Could you check a few things on this drawing? It's one solid part, dimensions in mm from its lowest x, y, z. A direction names the side the tool comes from. Give positions to 0.01 mm unless a question says otherwise; leave off trailing zeros. Loops run counter-clockwise (first coordinate to the right, second up) from the corner with the lowest first, then second, coordinate; pieces in that order, holes last.
Q1. Suppose I cut it at A-A (x = 35). List the corners of the cut face in (y, z) for me.
Q2. For the marked faces 5 and 6, which set-ups out of +Z, -Z, +X, -X, +Y, -Y let a thin tool reach every point of the face, with its end or its side?
Q3. I need wall thicknesses on probe 1 along X at (y, z) = (36, 17.5) (1 decimal); probe 2 along Y at (x, z) = (17, 25) (1 decimal); probe 3 along Z at (x, y) = (29, 62). Which ranges of each line are inside material? Lowest first, please.
Q4. I'm going to push flat-ended pins straight in: P1, Ø4, axis at x = 57, y = 52, coming from the +Z side; P2, Ø3, axis at y = 38, z = 49, coming from the -X side; P3, Ø12, axis at y = 51.5, z = 47.5, coming from the +X side (1 decimal). Where does each tip first touch, or does it pass through?
Q5. Suppose I cut it at B-B (y = 35). Count the separate pieces of the cut face and the enclosed holes in it, and give its area (3 significant figures).
Q6. Thinking about a two-plate mould opening in X: for the marked faces 1, 2, 3 and 4, which applies, pulls with the +X half, pulls with the -X half, needs draft (parallel to the pull), parting line crosses it, or undercut?
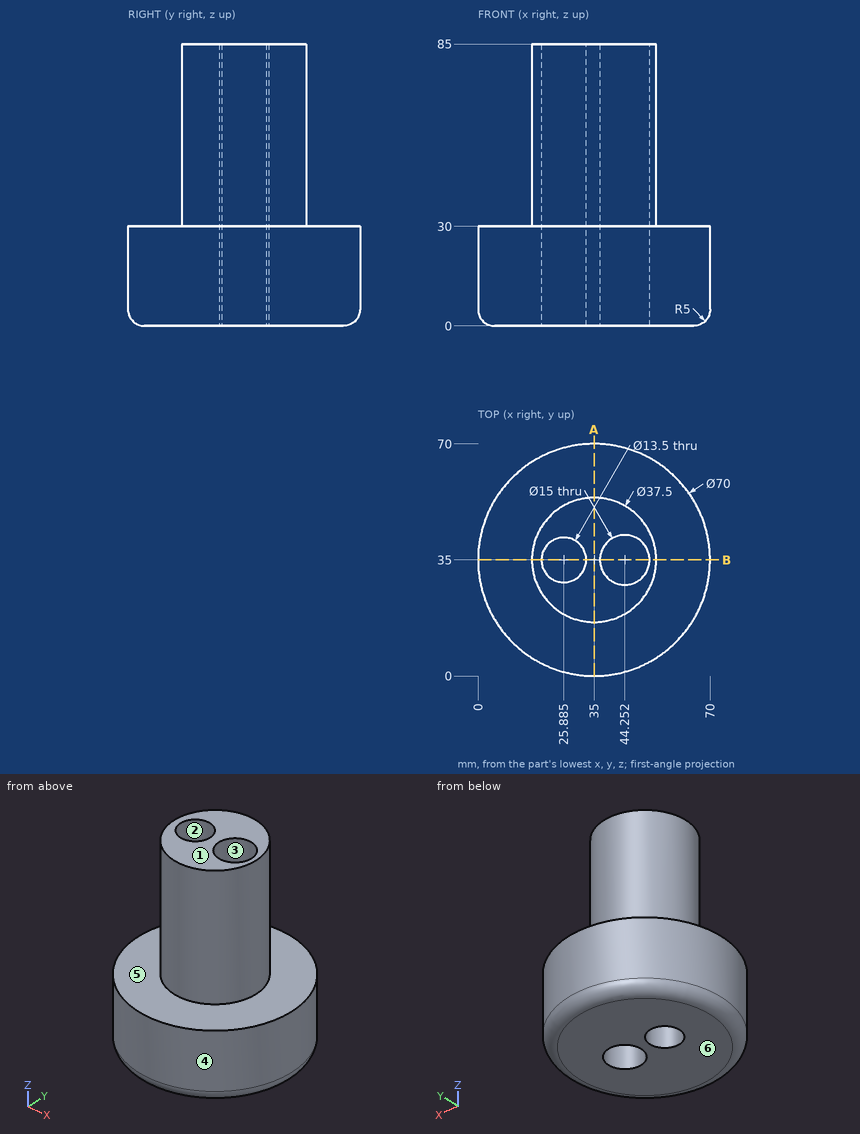
Solutions:
1. outline: (0, 5) arc R5 ccw to (5, 0) - (65, 0) arc R5 ccw to (70, 5) - (70, 30) - (53.75, 30) - (53.75, 85) - (16.25, 85) - (16.25, 30) - (0, 30) - close
2. face 5: +Z
2. face 6: -Z, +X, -X, +Y, -Y
3. probe 1: x = 0 to 19.2, 32.6 to 36.8, 51.7 to 70
3. probe 2: y = 5 to 65
3. probe 3: z = 0 to 30
4. P1: stops at z = 30
4. P2: stops at x = 16.31
4. P3: stops at x = 50.5
5. separate pieces: 3
5. enclosed holes: 0
5. area: 1,730 mm2
6. face 1: needs draft
6. face 2: undercut
6. face 3: undercut
6. face 4: parting line crosses it
